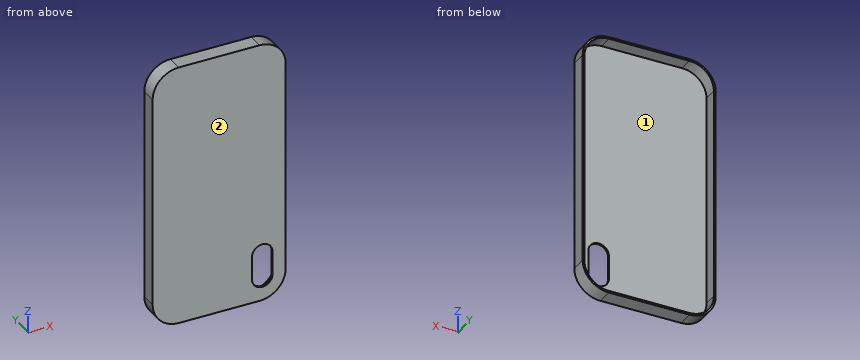
```python
from build123d import *

# Parameters (mm, degrees)
BOSS_EXTRUDE1_DEPTH = 8.7
CUT_EXTRUDE1_DEPTH  = 7.7
CUT_EXTRUDE2_DEPTH  = 2


with BuildPart() as part:
    # Sketch1 → Boss-Extrude1 (new body)
    with BuildSketch(Plane(origin=(0, 0, 0), x_dir=(1, 0, 0), z_dir=(0, 1, 0))):
        with BuildLine():
            Line((-22.08, -72.785), (22.08, -72.785))
            ThreePointArc((22.08, -72.785), (32.255266581, -68.570266581), (36.47, -58.395))
            Line((36.47, -58.395), (36.47, 58.395))
            ThreePointArc((36.47, 58.395), (32.255266581, 68.570266581), (22.08, 72.785))
            Line((22.08, 72.785), (-22.08, 72.785))
            ThreePointArc((-22.08, 72.785), (-32.255266581, 68.570266581), (-36.47, 58.395))
            Line((-36.47, 58.395), (-36.47, -58.395))
            ThreePointArc((-36.47, -58.395), (-32.255266581, -68.570266581), (-22.08, -72.785))
        make_face()
    extrude(amount=BOSS_EXTRUDE1_DEPTH)

    # Sketch2 → Cut-Extrude1 (cut)
    with BuildSketch(Plane(origin=(0, 8.7, 0), x_dir=(1, 0, 0), z_dir=(0, 1, 0))):
        with BuildLine():
            Line((-22.08, -71.785), (22.08, -71.785))
            ThreePointArc((22.08, -71.785), (31.5481598, -67.8631598), (35.47, -58.395))
            Line((35.47, -58.395), (35.47, 58.395))
            ThreePointArc((35.47, 58.395), (31.5481598, 67.8631598), (22.08, 71.785))
            Line((22.08, 71.785), (-22.08, 71.785))
            ThreePointArc((-22.08, 71.785), (-31.5481598, 67.8631598), (-35.47, 58.395))
            Line((-35.47, 58.395), (-35.47, -58.395))
            ThreePointArc((-35.47, -58.395), (-31.5481598, -67.8631598), (-22.08, -71.785))
        make_face()
    extrude(amount=-CUT_EXTRUDE1_DEPTH, mode=Mode.SUBTRACT)

    # Sketch3 → Cut-Extrude2 (cut, through all)
    with BuildSketch(Plane(origin=(0, 1, 0), x_dir=(1, 0, 0), z_dir=(0, 1, 0))):
        with BuildLine():
            Line((29.28, 59.6), (29.28, 46.63))
            ThreePointArc((29.28, 46.63), (23.65, 41), (18.02, 46.63))
            Line((18.02, 46.63), (18.02, 59.6))
            ThreePointArc((18.02, 59.6), (23.65, 65.23), (29.28, 59.6))
        make_face()
    extrude(amount=-CUT_EXTRUDE2_DEPTH, mode=Mode.SUBTRACT)


solid = part.part
```
CAD build for the part. Positions are in the model's coordinates, mm. Face numbers are marked on the shaded views. Round coordinates to 2 decimals unless told otherwise and drop trailing zeros. Order: outer loops, then holes, each group sorted by start corner. A loop starts at its lowest first (then second) coordinate and runs counter-clockwise, first axis right, second up.
Q1. Slice it at C-C (x = 12). Write the cut outline in (y, z) (3 decimals), and give its area (3 significant figures).
Q2. Two-plate mould, pull along Z, no slides. Class the marked faces 1 and 2: pulls with the +Z half, pulls with the -Z half, needs draft (parallel to the pull), parting line crosses it, or undercut.
Q3. Slice it at D-D (x = 23.65). Write the cut outline in (y, z).
Q4. Slice it at B-B (z = -12.5). Write the cut outline in (x, y), and give its area (3 significant figures).
Q5. Slice it at A-A (y = 2.5). Write the cut outline in (x, z) (3 decimals), and give its area (3 significant figures).
Q6. Wall check: L1, parallel to Z at x = -21, y = 4 (3 decimals); L2, parallel to X at y = 7.5, z = -58; L3, parallel to Y at x = -32.5, z = 42. Give the ranges that are in metal, low to high.
Q7. Drop a flat-ended pin along its axis: pin 1 (12 mm diameter, centred on x = -16.5, z = 25.5, fed in from +Y). Give the stop position or say it passes through.
Results below:
1. outline: (0, -72.785) - (8.7, -72.785) - (8.7, -71.785) - (1, -71.785) - (1, 71.785) - (8.7, 71.785) - (8.7, 72.785) - (0, 72.785) - close
1. area: 161 mm2
2. face 1: undercut
2. face 2: needs draft
3. outline: (0, -72.7) - (8.7, -72.7) - (8.7, -71.69) - (1, -71.69) - (1, -65.23) - (0, -65.23) - close; (0, -41) - (1, -41) - (1, 71.69) - (8.7, 71.69) - (8.7, 72.7) - (0, 72.7) - close
4. outline: (-36.47, 0) - (36.47, 0) - (36.47, 8.7) - (35.47, 8.7) - (35.47, 1) - (-35.47, 1) - (-35.47, 8.7) - (-36.47, 8.7) - close
4. area: 88.3 mm2
5. outline: (-36.47, -58.395) arc R14.39 ccw to (-22.08, -72.785) - (22.08, -72.785) arc R14.39 ccw to (36.47, -58.395) - (36.47, 58.395) arc R14.39 ccw to (22.08, 72.785) - (-22.08, 72.785) arc R14.39 ccw to (-36.47, 58.395) - close; hole (-35.47, -58.395) arc R13.39 ccw to (-22.08, -71.785) - (22.08, -71.785) arc R13.39 ccw to (35.47, -58.395) - (35.47, 58.395) arc R13.39 ccw to (22.08, 71.785) - (-22.08, 71.785) arc R13.39 ccw to (-35.47, 58.395) - close
5. area: 409 mm2
6. L1: z = -72.785 to -71.785, 71.785 to 72.785
6. L2: x = -36.47 to -35.47, 35.47 to 36.47
6. L3: y = 0 to 1
7. pin 1: stops at y = 1
